The listing builds one solid part. Answer for the finished solid, in the listing's coordinates (mm). A direction names the side the tool comes from. Round coordinates to 2 decimals unless told otherwise and drop trailing zeros. Loops run counter-clockwise (first coordinate to the right, second up) from the corner with the lowest first, then second, coordinate; pieces in that order, holes last. Notation, with made-up numbers: (-7, 76.25) - (41, 76.25) arc R5 ccw to (41, 83.25) - close; hole circle Ø10 at (-33, 56). An arc over 180 degrees is marked (long way). One line per item, written item: value.
```python
from build123d import *

# Parameters (mm, degrees)
SALIENTE_EXTRUIR1_DEPTH = 3


with BuildPart() as part:
    # Croquis1 → Saliente-Extruir1 (new body)
    with BuildSketch(Plane.XY):
        with BuildLine():
            Line((-2.649110641, 0), (-15, 0))
            ThreePointArc((-15, 0), (-18.535533906, -1.464466094), (-20, -5))
            Line((-20, -5), (-20, -10))
            Line((-20, -10), (-15.546822742, -10))
            Line((-15.546822742, -10), (-15.546822742, -16))
            Line((-15.546822742, -16), (14.453177258, -16))
            Line((14.453177258, -16), (14.453177258, -10))
            Line((14.453177258, -10), (20, -10))
            Line((20, -10), (20, 0))
            ThreePointArc((20, 0), (11.161711866, 9.932292059), (0.269914892, 2.307692308))
            ThreePointArc((0.269914892, 2.307692308), (-0.788589622, 0.646606378), (-2.649110641, 0))
        make_face()
        with BuildLine():
            Line((-15.546822742, -6.391304348), (12.453177258, -6.391304348))
            ThreePointArc((12.453177258, -6.391304348), (13.86739082, -5.80551791), (14.453177258, -4.391304348))
            Line((14.453177258, -4.391304348), (14.453177258, -3.391304348))
            Line((14.453177258, -3.391304348), (14.453177258, 1.869565217))
            ThreePointArc((14.453177258, 1.869565217), (13.574497601, 3.990885561), (11.453177258, 4.869565217))
            Line((11.453177258, 4.869565217), (9.93812709, 4.869565217))
            ThreePointArc((9.93812709, 4.869565217), (7.816806747, 3.990885561), (6.93812709, 1.869565217))
            Line((6.93812709, 1.869565217), (6.93812709, -1.391304348))
            ThreePointArc((6.93812709, -1.391304348), (6.352340653, -2.80551791), (4.93812709, -3.391304348))
            Line((4.93812709, -3.391304348), (-15.546822742, -3.391304348))
            Line((-15.546822742, -3.391304348), (-15.546822742, -6.391304348))
        make_face(mode=Mode.SUBTRACT)
    extrude(amount=SALIENTE_EXTRUIR1_DEPTH)


solid = part.part
```
1) Each of these flat-tipped pins is pushed along its axis until it touches: pin 1 Ø1.5 at (x, z) = (-18.5, 1) entering from -Y; pin 2 Ø1.5 at (y, z) = (-13, 1) entering from +X; pin 3 Ø1.5 at (x, y) = (-13, -4.5) entering from +Z; pin 4 Ø4 at (x, y) = (1, -5.5) entering from +Z. Where does it stop, or does it pass through?
Final values:
pin 1: y = -10
pin 2: x = 14.45
pin 3: through
pin 4: z = 3
2) A cutting plane is placed at B-B on z = 0.4. Give the vertices of the cut face in (x, y), and give its area (3 significant figures).
Final values:
outline: (-20, -10) - (-15.55, -10) - (-15.55, -16) - (14.45, -16) - (14.45, -10) - (20, -10) - (20, 0) arc R10 ccw to (0.27, 2.31) arc R3 cw to (-2.65, 0) - (-15, 0) arc R5 ccw to (-20, -5) - close; hole (-15.55, -6.39) - (12.45, -6.39) arc R2 ccw to (14.45, -4.39) - (14.45, 1.87) arc R3 ccw to (11.45, 4.87) - (9.94, 4.87) arc R3 ccw to (6.94, 1.87) - (6.94, -1.39) arc R2 cw to (4.94, -3.39) - (-15.55, -3.39) - close
area: 585 mm2
3) A cutting plane is placed at D-D on y = -11.5. Give the vertices of the cut face in (x, z), and give its area (3 significant figures).
Final values:
outline: (-15.55, 0) - (14.45, 0) - (14.45, 3) - (-15.55, 3) - close
area: 90.0 mm2
4) Consider L1, parallel to Y at x = -8, z = 0.85; L2, parallel to Y at x = 10, z = 2.2; L3, parallel to X at y = -11, z = 2.4. Determine where each line is inside the solid, lowest interval first.
Final values:
L1: -16 to -6.39, -3.39 to 0
L2: -16 to -6.39, 4.87 to 10
L3: -15.55 to 14.45
5) A cutting plane is placed at A-A on x = -14.5. Give the vertices of the cut face in (y, z).
Final values:
outline: (-16, 0) - (-6.39, 0) - (-6.39, 3) - (-16, 3) - close; (-3.39, 0) - (0, 0) - (0, 3) - (-3.39, 3) - close
6) A cutting plane is placed at C-C on y = -2.25. Give the vertices of the cut face in (x, z).
Final values:
outline: (-19.18, 0) - (6.74, 0) - (6.74, 3) - (-19.18, 3) - close; (14.45, 0) - (20, 0) - (20, 3) - (14.45, 3) - close
7) For a pull along Y with two mould halves and no side action, classify faces 1 (the flat face through (-9, 0, 1)), 2 (the flat face through (-1, -16, 1)), 3 (the flat face through (0, -3, 0)), 4 (the flat face through (11, 4.87, 1)) as released by +Y, released by -Y, zero draft, split by the parting line, or undercut.
Final values:
face 1: released by +Y
face 2: released by -Y
face 3: zero draft
face 4: undercut
8) For faces 5 (the flat face through (17, -10, 1)), 6 (the flat face through (-5, -3.391, 1)), 7 (the cylindrical face through (-0.77, 0.66, 1.48)), 8 (the cylindrical face through (11.4, 9.9, 1.5)), 9 (the flat face through (-18, -10, 1)), determine the directions among +Z, -Z, +X, -X, +Y, -Y from which every point of the face is accessible in a straight line to the end or side of a thin tool.
Final values:
face 5: +Z, -Z, +X, -Y
face 6: +Z, -Z
face 7: +Z, -Z, -X, +Y
face 8: +Z, -Z, +Y
face 9: +Z, -Z, -X, -Y
